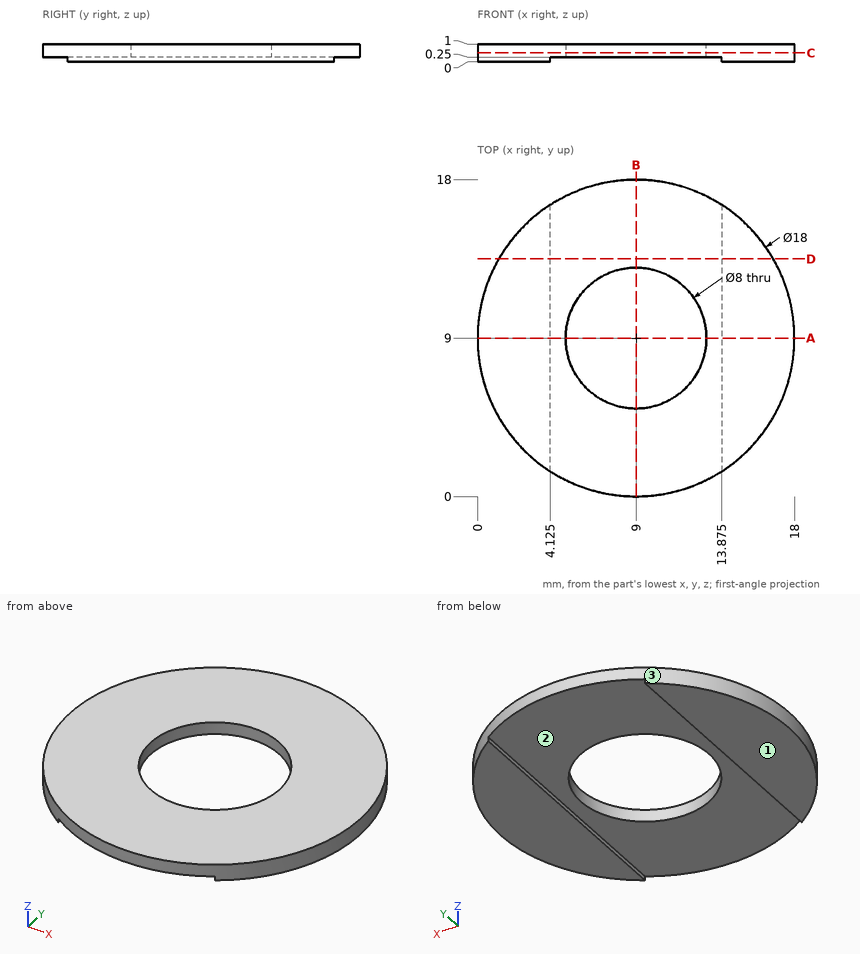
Here's the drawing with two shaded views (mm, measured from the low corner). I have some questions. Round coordinates to 2 decimals unless told otherwise and drop trailing zeros. Order: outer loops, then holes, each group sorted by start corner. A loop starts at its lowest first (then second) coordinate and runs counter-clockwise, first axis right, second up. Notation, with made-up numbers: M 13,60 L 70,60 A19 cw 70,70 Z; hole C 39,-34.75 d9. An arc over 180 degrees is marked long. Use CSV: the item, a comma, the result in double quotes.
1) I'm going to push flat-ended pins straight in: P1, Ø9, axis at x = 9, y = 9, coming from the +Z side; P2, Ø5, axis at x = 7.5, y = 5, coming from the -Z side. Where does each tip first touch, or does it pass through?
Taken from the geometry:
P1,"z = 1"
P2,"z = 0.25"
2) I want a section at A-A (y = 9). List the corners of the cut face in (x, z) for me (3 decimals), then the cut area to 3 significant figures.
Taken from the geometry:
outline,"M 0,0 L 4.125,0 L 4.125,0.25 L 5,0.25 L 5,1 L 0,1 Z; M 13,0.25 L 13.875,0.25 L 13.875,0 L 18,0 L 18,1 L 13,1 Z"
area,"9.56 mm^2"
3) I want a section at D-D (y = 13.5). List the corners of the cut face in (x, z) for me (3 decimals).
Taken from the geometry:
outline,"M 1.206,0 L 4.125,0 L 4.125,0.25 L 13.875,0.25 L 13.875,0 L 16.794,0 L 16.794,1 L 1.206,1 Z"
4) I want a section at B-B (x = 9). List the corners of the cut face in (y, z) for me, then the cut area to 3 significant figures.
Taken from the geometry:
outline,"M 0,0.25 L 5,0.25 L 5,1 L 0,1 Z; M 13,0.25 L 18,0.25 L 18,1 L 13,1 Z"
area,"7.50 mm^2"
5) I want a section at C-C (z = 0.5). List the corners of the cut face in (x, y) for me.
Taken from the geometry:
outline,"C 9,9 d18; hole C 9,9 d8"
6) I need wall thicknesses on line 1 along Y through (x, z) = (9, 0.75); line 2 along Z through (x, y) = (9, 3). Which ranges of each line are inside material? Lowest first, please. Write a range as [from, to].
Taken from the geometry:
line 1,"[0, 5], [13, 18]"
line 2,"[0.25, 1]"
7) If we mould it in two halves opening along X, with no side actions, what happens to the marked faces 1, 2 and 3? For each: pulls with the +X half, pulls with the -X half, needs draft (parallel to the pull), parting line crosses it, or undercut.
Taken from the geometry:
face 1,"needs draft"
face 2,"undercut"
face 3,"parting line crosses it"
